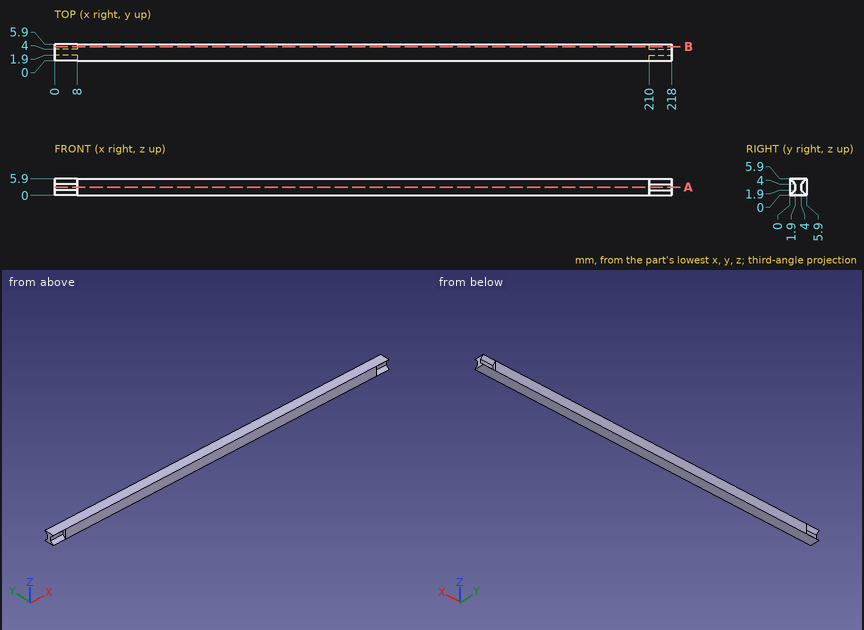
The figure shows three views and two pictorial views of one solid part (mm, origin at its lowest corner). Answer the questions. Round coordinates to 2 decimals unless told otherwise and drop trailing zeros. Write each loop counter-clockwise with the first axis right and the second up, starting at its lowest first coordinate (ties: lowest second). Pieces come first, ordered by that corner, then holes. Notation, with made-up numbers: (43.5, 39.5) - (80.5, 39.5) arc R19 cw to (80.5, 59.5) - close; hole circle Ø11 at (69.5, -1). An arc over 180 degrees is marked (long way). Answer in a Markdown table with one row per item. Add a question column.
1. A cutting plane is placed at B-B, the plane y = 4.95. Determine the outline of the cut face in (x, z).
2. Given pin 1 (1 mm diameter, centred on y = 0.5, z = 3.5, fed in from +X); pin 2 (1.7 mm diameter, centred on x = 3, z = 3.5, fed in from -Y); pin 3 (1 mm diameter, centred on y = 1, z = 3, fed in from -X), each flat-ended and moving along its own axis, determine where each tip first touches the part or whether it passes through.
3. Find the intervals of material crossed by line 1 along X through (y, z) = (1.65, 3.75), in increasing order. Write a range as from..to.
4. A cutting plane is placed at A-A, the plane z = 2.9. Determine the outline of the cut face in (x, y).
Worked out:
| question | item | result |
|---|---|---|
| 1 | outline | (0, 0) - (218, 0) - (218, 0.95) - (210, 0.95) - (210, 4.95) - (218, 4.95) - (218, 5.9) - (0, 5.9) - (0, 4.95) - (8, 4.95) - (8, 0.95) - (0, 0.95) - close |
| 2 | pin 1 | x = 210 |
| 2 | pin 2 | y = 1.55 |
| 2 | pin 3 | x = 8 |
| 3 | line 1 | 8..210 |
| 4 | outline | (0, 1.9) - (8, 1.9) - (8, 0) - (210, 0) - (210, 1.9) - (218, 1.9) - (218, 4) - (210, 4) - (210, 5.9) - (8, 5.9) - (8, 4) - (0, 4) - close |
